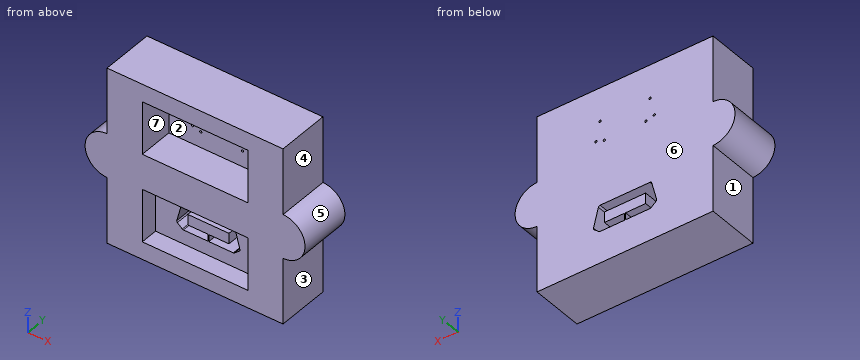
```python
from build123d import *

# Parameters (mm, degrees)
BOSS_EXTRUDE1_DEPTH = 30
CUT_EXTRUDE2_DEPTH  = 20
SKETCH3_R           = 0.625
CUT_EXTRUDE3_DEPTH  = 10
SKETCH4_W           = 60
SKETCH4_H           = 30
CUT_EXTRUDE4_DEPTH  = 10
SKETCH5_W           = 60
SKETCH5_H           = 30
CUT_EXTRUDE5_DEPTH  = 20


with BuildPart() as part:
    # Sketch2 → Boss-Extrude1 (new body)
    with BuildSketch(Plane(origin=(0, 0, 0), x_dir=(1, 0, 0), z_dir=(0, 1, 0))):
        with BuildLine():
            Line((-50, -75), (50, -75))
            Line((50, -75), (50, -37.5))
            ThreePointArc((50, -37.5), (62.5, -25), (50, -12.5))
            Line((50, -12.5), (50, 25))
            Line((50, 25), (-50, 25))
            Line((-50, 25), (-50, -12.5))
            ThreePointArc((-50, -12.5), (-62.5, -25), (-50, -37.5))
            Line((-50, -37.5), (-50, -75))
        make_face()
    extrude(amount=-BOSS_EXTRUDE1_DEPTH)

    # Sketch1 → Cut-Extrude2 (cut)
    with BuildSketch(Plane(origin=(0, 0, 0), x_dir=(1, 0, 0), z_dir=(0, 1, 0))):
        with BuildLine():
            Line((-14.178620776, -8), (14.178620776, -8))
            ThreePointArc((14.178620776, -8), (14.789399734, -7.791801152), (15.145851741, -7.253898128))
            Line((15.145851741, -7.253898128), (17.939776994, 3.389626646))
            ThreePointArc((17.939776994, 3.389626646), (17.926022481, 3.944992277), (17.618005902, 4.407318956))
            Line((17.618005902, 4.407318956), (14.829510217, 6.763794182))
            ThreePointArc((14.829510217, 6.763794182), (14.527711383, 6.939093761), (14.184050345, 7))
            Line((14.184050345, 7), (0.25, 7))
            Line((0.25, 7), (0.25, 3))
            Line((0.25, 3), (11.7, 3))
            Line((11.7, 3), (11.7, -3))
            Line((11.7, -3), (-11.7, -3))
            Line((-11.7, -3), (-11.7, 3))
            Line((-11.7, 3), (-0.25, 3))
            Line((-0.25, 3), (-0.25, 7))
            Line((-0.25, 7), (-14.184050345, 7))
            ThreePointArc((-14.184050345, 7), (-14.527711383, 6.939093761), (-14.829510217, 6.763794182))
            Line((-14.829510217, 6.763794182), (-17.618005902, 4.407318956))
            ThreePointArc((-17.618005902, 4.407318956), (-17.926022481, 3.944992277), (-17.939776994, 3.389626646))
            Line((-17.939776994, 3.389626646), (-15.145851741, -7.253898128))
            ThreePointArc((-15.145851741, -7.253898128), (-14.789399734, -7.791801152), (-14.178620776, -8))
        make_face()
    extrude(amount=-CUT_EXTRUDE2_DEPTH, mode=Mode.SUBTRACT)

    # Sketch3 → Cut-Extrude3 (cut)
    with BuildSketch(Plane(origin=(0, 0, 0), x_dir=(1, 0, 0), z_dir=(0, 1, 0))):
        with Locations((-14.217473576, -55.961496156)):
            Circle(SKETCH3_R)
        with Locations((14.182526424, -55.961496156)):
            Circle(SKETCH3_R)
        with Locations((-16.617473576, -45.317971382)):
            Circle(SKETCH3_R)
        with Locations((16.582526424, -45.317971382)):
            Circle(SKETCH3_R)
        with Locations((-11.867473576, -43.961496156)):
            Circle(SKETCH3_R)
        with Locations((11.832526424, -43.961496156)):
            Circle(SKETCH3_R)
    extrude(amount=-CUT_EXTRUDE3_DEPTH, mode=Mode.SUBTRACT)

    # Sketch4 → Cut-Extrude4 (cut)
    with BuildSketch(Plane.XZ.offset(30)):
        Rectangle(SKETCH4_W, SKETCH4_H)
    extrude(amount=-CUT_EXTRUDE4_DEPTH, mode=Mode.SUBTRACT)

    # Sketch5 → Cut-Extrude5 (cut)
    with BuildSketch(Plane.XZ.offset(30)):
        with Locations((0, 50)):
            Rectangle(SKETCH5_W, SKETCH5_H)
    extrude(amount=-CUT_EXTRUDE5_DEPTH, mode=Mode.SUBTRACT)


solid = part.part
```
Build history of the part. All positions in model axes, mm. Face numbers are marked on the shaded views. A direction names the side the tool comes from. Round coordinates to 2 decimals unless told otherwise and drop trailing zeros. Loops run counter-clockwise (first coordinate to the right, second up) from the corner with the lowest first, then second, coordinate; pieces in that order, holes last.
Item 1: Saw through at D-D (z = -1.5). List the corners of the cut face in (x, y).
Item 2: Pin check, flat tips, straight feed: P1, Ø4.5, axis at y = -7.5, z = -4.5, coming from the +X side; P2, Ø10, axis at y = -17, z = -11, coming from the -X side; P3, Ø1.6, axis at x = -11.87, z = 43.96, coming from the -Y side; P4, Ø1, axis at x = -14.22, z = 55.96, coming from the -Y side. Stop position of each tip, or through.
Item 3: Which spindle directions (+Z, -Z, +X, -X, +Y, -Y) get a long thin tool onto all of the face, cutting with end or side? Do the marked faces 1, 2, 3 and 4. Say none if no direction does.
Item 4: Saw through at C-C (x = 28). List the corners of the cut face in (y, z).
Item 5: Saw through at B-B (z = 59.5). List the corners of the cut face in (x, y), then the cut area to 3 significant figures.
Item 6: Saw through at A-A (y = -21.75). List the corners of the cut face in (x, z).
Item 7: Two-plate mould, pull along X, no slides. Class the marked faces 5, 6 and 7: released by +X, released by -X, zero draft, split by the parting line, or undercut.
Item 8: Drill centre lines: line 1 along Z through (x, y) = (-11, -25); line 2 along X through (y, z) = (-19.25, 57.5); line 3 along Z through (x, y) = (5, -18). Where is each one in solid material? Low to high.
Worked answers:
1. outline: (-50, -30) - (-30, -30) - (-30, -20) - (-17.44, -20) - (-17.44, 0) - (-50, 0) - close; (-11.7, -20) - (11.7, -20) - (11.7, 0) - (-11.7, 0) - close; (17.44, -20) - (30, -20) - (30, -30) - (50, -30) - (50, 0) - (17.44, 0) - close
2. P1: stops at x = 50
2. P2: stops at x = -50
2. P3: stops at y = -10
2. P4: passes through
3. face 1: -Z, -X, +Y, -Y
3. face 2: -Y
3. face 3: -Z, +X, +Y, -Y
3. face 4: +Z, +X, +Y, -Y
4. outline: (-30, -25) - (0, -25) - (0, 75) - (-30, 75) - (-30, 65) - (-10, 65) - (-10, 35) - (-30, 35) - (-30, 15) - (-20, 15) - (-20, -15) - (-30, -15) - close
5. outline: (-50, -30) - (-30, -30) - (-30, -10) - (30, -10) - (30, -30) - (50, -30) - (50, 0) - (-50, 0) - close
5. area: 1,800 mm2
6. outline: (-50, -25) - (50, -25) - (50, 12.5) arc R12.5 ccw to (50, 37.5) - (50, 75) - (-50, 75) - (-50, 37.5) arc R12.5 ccw to (-50, 12.5) - close; hole (-30, -15) - (30, -15) - (30, 15) - (-30, 15) - close; hole (-30, 35) - (30, 35) - (30, 65) - (-30, 65) - close
7. face 5: released by +X
7. face 6: zero draft
7. face 7: undercut
8. line 1: z = -25 to -15, 15 to 35, 65 to 75
8. line 2: x = -50 to -30, 30 to 50
8. line 3: z = -25 to -7, -3 to 3, 8 to 35, 65 to 75
